Source: CAD feature listing. Evaluate the final solid. Frame: model axes, mm. Give positions to 0.01 mm unless a question says otherwise; leave off trailing zeros. Write each loop counter-clockwise with the first axis right and the second up, starting at its lowest first coordinate (ties: lowest second). Pieces come first, ordered by that corner, then holes. Notation, with made-up numbers: M 39,45 L 78,45 A24 cw 78,79 Z; hole C 79,72.5 d4. An arc over 180 degrees is marked long. Answer as a JSON object with one key per item and string values. Group by question number.
```python
from build123d import *

# Parameters (mm, degrees)
CROQUIS1_R               = 103.5
CROQUIS1_R_2             = 97.5
BASE_DEPTH               = 200
DISE_O_DEPTH             = 150
DISE_O_DEPTH_BACK        = 150
PATR_NTRASERO_DEPTH      = 20
PATR_NTRASERO_DEPTH_BACK = 90


with BuildPart() as part:
    # Croquis1 → Base (new body)
    with BuildSketch(Plane.XY):
        Circle(CROQUIS1_R)
        Circle(CROQUIS1_R_2, mode=Mode.SUBTRACT)
    extrude(amount=BASE_DEPTH)

    # Croquis2 → Diseño (cut, two sides)
    with BuildSketch(Plane(origin=(0, 0, 0), x_dir=(1, 0, 0), z_dir=(0, 1, 0))) as dise_o_sk:
        Polygon((-103.5, 0), (-103.5, -200), (-72.714481971, -78.691726895), (-45.812787176, -141.817485969), (0, 0), align=None)
        Polygon((72.714481971, -78.691726895), (103.5, -200), (103.5, 0), (0, 0), (45.812787176, -141.817485969), align=None)
    extrude(amount=DISE_O_DEPTH, mode=Mode.SUBTRACT)
    extrude(dise_o_sk.sketch, amount=-DISE_O_DEPTH_BACK, mode=Mode.SUBTRACT)

    # Croquis12 → PatrónTrasero (cut, two sides)
    with BuildSketch(Plane(origin=(0, -90, 0), x_dir=(-1, 0, 0), z_dir=(0, -1, 0))) as patr_ntrasero_sk:
        Polygon((-103.5, 1.909548239), (-103.5, -200), (-79.959810945, -107.241460736), (-45.812787176, -145.013726935), (0, -76.028192757), (45.812787176, -145.013726935), (79.959810945, -107.241460736), (103.5, -200), (103.5, 1.909548239), align=None)
    extrude(amount=PATR_NTRASERO_DEPTH, mode=Mode.SUBTRACT)
    extrude(patr_ntrasero_sk.sketch, amount=-PATR_NTRASERO_DEPTH_BACK, mode=Mode.SUBTRACT)

    # Croquis14 → RanuraPrimalJewel section 0
    with BuildSketch(Plane(origin=(0, 103.5, 0), x_dir=(1, 0, 0), z_dir=(0, 1, 0))):
        Polygon((15, -165), (15, -125), (0, -105), (-15, -125), (-15, -165), (0, -185), align=None)
    # Croquis17 → RanuraPrimalJewel section 1
    with BuildSketch(Plane(origin=(0, 94.5, 0), x_dir=(1, 0, 0), z_dir=(0, 1, 0))):
        Polygon((-9, -127), (0, -115), (9, -127), (9, -163), (0, -175), (-9, -163), align=None)
    loft(mode=Mode.SUBTRACT)

    # Croquis20 → Cortar-Recubrir1 section 0
    with BuildSketch(Plane(origin=(-65.973382939, 79.748120627, 0), x_dir=(0, 0, 1), z_dir=(-0.63742399, 0.770513243, 0))):
        Polygon((146.644660941, -9.078894023), (164.32233047, -26.756563553), (182, -9.078894023), (164.32233047, 8.598775507), align=None)
    # Croquis22 → Cortar-Recubrir1 section 1
    with BuildSketch(Plane(origin=(-60.236567031, 72.813501442, 0), x_dir=(0, 0, 1), z_dir=(-0.63742399, 0.770513243, 0))):
        Polygon((157.95836944, -9.078894023), (164.32233047, -15.442855054), (170.686291501, -9.078894023), (164.32233047, -2.714932992), align=None)
    loft(mode=Mode.SUBTRACT)

    # Croquis30 → Cortar-Recubrir2 section 0
    with BuildSketch(Plane(origin=(60.236567031, 72.813501442, 0), x_dir=(0, 0, 1), z_dir=(0.63742399, 0.770513243, 0))):
        Polygon((157.95836944, 9.078894023), (164.32233047, 2.714932992), (170.686291501, 9.078894023), (164.32233047, 15.442855054), align=None)
    # Croquis29 → Cortar-Recubrir2 section 1
    with BuildSketch(Plane(origin=(65.973382939, 79.748120627, 0), x_dir=(0, 0, 1), z_dir=(0.63742399, 0.770513243, 0))):
        Polygon((182, 9.078894023), (164.32233047, 26.756563553), (146.644660941, 9.078894023), (164.32233047, -8.598775507), align=None)
    loft(mode=Mode.SUBTRACT)


solid = part.part
```
(1) Section B-B, the plane x = -31. Return loops of the section in (y, z).
(2) Section D-D, the plane z = 19.5. Return loops of the section in (x, y).
(3) Pull-direction query (X, two-part tool) for faces 1 (the flat face through (-64.07, -75.76, 124.82)), 2 (the flat face through (96.017, 19.129, 170.513)), 3 (the flat face through (-97.3, 8.81, 175.57)); classes: pulls with the +X half, pulls with the -X half, needs draft (parallel to the pull), parting line crosses it, or undercut.
(4) Section C-C, the plane y = 31.5. Return loops of the section in (x, z).
(5) Ray query, L1, parallel to Y at x = 0, z = 83; L2, parallel to Y at x = 0, z = 56; L3, parallel to Y at x = -44, z = 151. Return the intervals inside material, ascending. Write a range as [from, to].
(6) Section A-A, the plane z = 102. Return loops of the section in (x, y).
(7) Contact query for flat-ended pins moving along their axis: pin 1 Ø8 at (x, z) = (6, 101.5) entering from +Y; pin 2 Ø12 at (y, z) = (-61, 171) entering from +X; pin 3 Ø8 at (y, z) = (-82.5, 150.5) entering from +X. Output: stop coordinate, or through.
Reported:
{
 "1": {"outline": "M -98.75,122.71 L -92.44,122.71 L -92.44,200 L -98.75,200 Z; M 92.44,95.96 L 98.75,95.96 L 98.75,200 L 92.44,200 Z"},
 "2": {"outline": "M -6.3,97.3 A97.5 cw 6.3,97.3 L 6.3,103.31 A103.5 ccw -6.3,103.31 Z"},
 "3": {"face 1": "undercut", "face 2": "pulls with the +X half", "face 3": "pulls with the -X half"},
 "4": {"outline": "M -98.59,180.65 L -92.27,155.75 L -92.27,200 L -98.59,200 Z; M 92.27,155.75 L 98.59,180.65 L 98.59,200 L 92.27,200 Z"},
 "5": {"L1": "y = [-103.5, -97.5], [97.5, 103.5]", "L2": "y = [97.5, 103.5]", "L3": "y = [-93.68, -87.01], [87.01, 93.68]"},
 "6": {"outline": "M -78.63,57.65 A97.5 cw -62.78,74.6 L -62.78,82.28 A103.5 ccw -78.63,67.3 Z; M -32.95,91.76 A97.5 cw 32.95,91.76 L 32.95,98.11 A103.5 ccw -32.95,98.11 Z; M -17.25,-102.05 A103.5 ccw 17.25,-102.05 L 17.25,-95.96 A97.5 cw -17.25,-95.96 Z; M 62.78,74.6 A97.5 cw 78.63,57.65 L 78.63,67.3 A103.5 ccw 62.78,82.28 Z"},
 "7": {"pin 1": "stops at y = 103.48", "pin 2": "stops at x = 87.68", "pin 3": "stops at x = 67.45"}
}
